CAD build for the part. Positions are in the model's coordinates, mm. Coordinates: 2 decimals unless noted, no trailing zeros. Loops run counter-clockwise (first coordinate to the right, second up) from the corner with the lowest first, then second, coordinate; pieces in that order, holes last.
1) Saw through at A-A, the plane y = 0. Write the cut outline in (x, z), and give its area (3 significant figures).
2) Saw through at B-B, the plane x = 0. Write the cut outline in (y, z).
3) Pin check, flat tips, straight feed: pin 1 Ø5 at (x, y) = (0, 0) entering from -Z; pin 2 Ø0.5 at (x, z) = (9.5, 506) entering from +Y; pin 3 Ø5 at (x, z) = (0.5, 195.5) entering from +Y; pin 4 Ø2.5 at (y, z) = (-1.5, 6) entering from +X. Stop position of each tip, or through.
4) Wall check: line 1 along Y through (x, z) = (-3.25, 277.5); line 2 along Z through (x, y) = (-3.5, -3). Give the ranges that are in metal, low to high.
```python
from build123d import *

# Parameters (mm, degrees)
SKETCH1_R               = 3.1
BOSS_EXTRUDE1_DEPTH     = 510
SKETCH3_R               = 4.5
CUT_EXTRUDE2_DEPTH      = 5.507107651
CUT_EXTRUDE2_DEPTH_BACK = 11


with BuildPart() as part:
    # Sketch1 → Boss-Extrude1 (new body)
    with BuildSketch(Plane.XY):
        with BuildLine():
            Line((-10, 3.1), (-8.2, 3.1))
            Line((-8.2, 3.1), (-8.2, 5.1))
            Line((-8.2, 5.1), (-6.4, 5.1))
            Line((-6.4, 5.1), (-5.492892349, 4.192892349))
            Line((-5.492892349, 4.192892349), (-5.492892349, -4.192892349))
            Line((-5.492892349, -4.192892349), (-6.4, -5.1))
            Line((-6.4, -5.1), (-8.2, -5.1))
            Line((-8.2, -5.1), (-8.2, -3.1))
            Line((-8.2, -3.1), (-10, -3.1))
            Line((-10, -3.1), (-10, -8.5))
            ThreePointArc((-10, -8.5), (-9.560660172, -9.560660172), (-8.5, -10))
            Line((-8.5, -10), (-3.1, -10))
            Line((-3.1, -10), (-3.1, -8.2))
            Line((-3.1, -8.2), (-5.1, -8.2))
            Line((-5.1, -8.2), (-5.1, -6.4))
            Line((-5.1, -6.4), (-4.192892349, -5.492892349))
            Line((-4.192892349, -5.492892349), (4.192892349, -5.492892349))
            Line((4.192892349, -5.492892349), (5.1, -6.4))
            Line((5.1, -6.4), (5.1, -8.2))
            Line((5.1, -8.2), (3.1, -8.2))
            Line((3.1, -8.2), (3.1, -10))
            Line((3.1, -10), (8.5, -10))
            ThreePointArc((8.5, -10), (9.560660172, -9.560660172), (10, -8.5))
            Line((10, -8.5), (10, -3.1))
            Line((10, -3.1), (8.2, -3.1))
            Line((8.2, -3.1), (8.2, -5.1))
            Line((8.2, -5.1), (6.4, -5.1))
            Line((6.4, -5.1), (5.492892349, -4.192892349))
            Line((5.492892349, -4.192892349), (5.492892349, 4.192892349))
            Line((5.492892349, 4.192892349), (6.4, 5.1))
            Line((6.4, 5.1), (8.2, 5.1))
            Line((8.2, 5.1), (8.2, 3.1))
            Line((8.2, 3.1), (10, 3.1))
            Line((10, 3.1), (10, 8.5))
            ThreePointArc((10, 8.5), (9.560660172, 9.560660172), (8.5, 10))
            Line((8.5, 10), (3.1, 10))
            Line((3.1, 10), (3.1, 8.2))
            Line((3.1, 8.2), (5.1, 8.2))
            Line((5.1, 8.2), (5.1, 6.4))
            Line((5.1, 6.4), (4.192892349, 5.492892349))
            Line((4.192892349, 5.492892349), (-4.192892349, 5.492892349))
            Line((-4.192892349, 5.492892349), (-5.1, 6.4))
            Line((-5.1, 6.4), (-5.1, 8.2))
            Line((-5.1, 8.2), (-3.1, 8.2))
            Line((-3.1, 8.2), (-3.1, 10))
            Line((-3.1, 10), (-8.5, 10))
            ThreePointArc((-8.5, 10), (-9.560660172, 9.560660172), (-10, 8.5))
            Line((-10, 8.5), (-10, 3.1))
        make_face()
        Circle(SKETCH1_R, mode=Mode.SUBTRACT)
    extrude(amount=BOSS_EXTRUDE1_DEPTH)

    # Sketch3 → Cut-Extrude2 (cut, two sides)
    with BuildSketch(Plane(origin=(5.492892349, 0, 0), x_dir=(0, 0, -1), z_dir=(1, 0, 0))) as cut_extrude2_sk:
        with Locations((-10, 0)):
            Circle(SKETCH3_R)
        with Locations((-500, 0)):
            Circle(SKETCH3_R)
    extrude(amount=CUT_EXTRUDE2_DEPTH, mode=Mode.SUBTRACT)
    extrude(cut_extrude2_sk.sketch, amount=-CUT_EXTRUDE2_DEPTH_BACK, mode=Mode.SUBTRACT)


solid = part.part
```
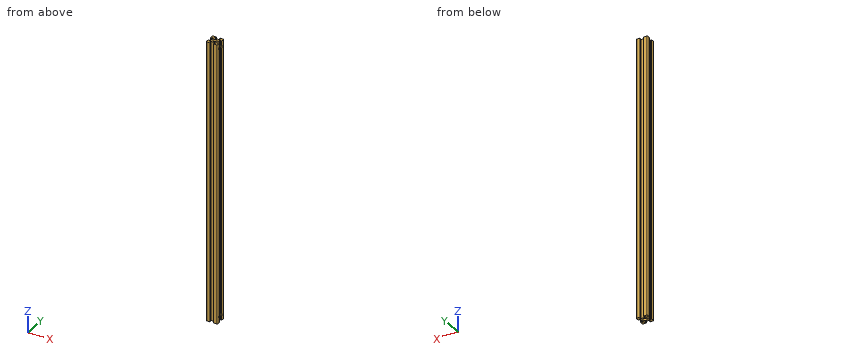
Data:
1. outline: (-5.49, 0) - (-3.1, 0) - (-3.1, 5.5) - (-5.49, 5.5) - close; (-5.49, 14.5) - (-3.1, 14.5) - (-3.1, 495.5) - (-5.49, 495.5) - close; (-5.49, 504.5) - (-3.1, 504.5) - (-3.1, 510) - (-5.49, 510) - close; (3.1, 0) - (5.49, 0) - (5.49, 5.5) - (3.1, 5.5) - close; (3.1, 14.5) - (5.49, 14.5) - (5.49, 495.5) - (3.1, 495.5) - close; (3.1, 504.5) - (5.49, 504.5) - (5.49, 510) - (3.1, 510) - close
1. area: 2,350 mm2
2. outline: (-5.49, 0) - (-3.1, 0) - (-3.1, 6.74) arc R4.5 cw to (-3.1, 13.26) - (-3.1, 496.74) arc R4.5 cw to (-3.1, 503.26) - (-3.1, 510) - (-5.49, 510) - close; (3.1, 0) - (5.49, 0) - (5.49, 510) - (3.1, 510) - (3.1, 503.26) arc R4.5 cw to (3.1, 496.74) - (3.1, 13.26) arc R4.5 cw to (3.1, 6.74) - close
3. pin 1: passes through
3. pin 2: stops at y = 9.8
3. pin 3: stops at y = 5.49
3. pin 4: stops at x = 5.49
4. line 1: y = -10 to -8.2, -5.49 to 5.49, 8.2 to 10
4. line 2: z = 0 to 6.65, 13.35 to 496.65, 503.35 to 510
